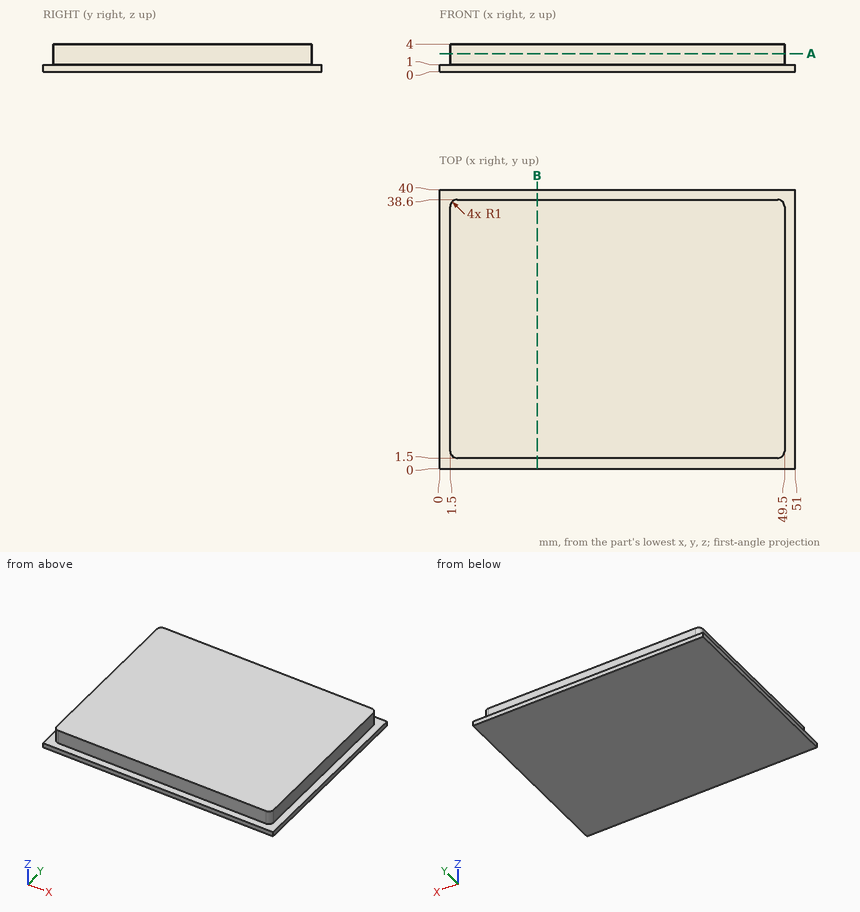
Answer from the drawing. Dimensions are ordinates in mm from the lowest x, y and z of the part. Coordinates: 2 decimals unless noted, no trailing zeros. Loops run counter-clockwise (first coordinate to the right, second up) from the corner with the lowest first, then second, coordinate; pieces in that order, holes last. Notation, with made-up numbers: (22.5, 64.25) - (67.5, 64.25) arc R21 cw to (67.5, 71.25) - close; hole circle Ø6 at (-10.75, -19). An arc over 180 degrees is marked (long way). Use a Markdown table: item, result.
Item 1: Consider probe 1 along X at (y, z) = (13, 2.8); probe 2 along Y at (x, z) = (18, 1.25). Determine where each line is inside the solid, lowest interval first. Write a range as from..to.
Evaluation:
| item | result |
|---|---|
| probe 1 | x = 1.5..49.5 |
| probe 2 | y = 1.5..38.6 |
Item 2: Find section A-A, the plane z = 2.6. Determine the outline of the cut face in (x, y), and give its area (3 significant figures).
Evaluation:
| item | result |
|---|---|
| outline | (1.5, 2.5) arc R1 ccw to (2.5, 1.5) - (48.5, 1.5) arc R1 ccw to (49.5, 2.5) - (49.5, 37.6) arc R1 ccw to (48.5, 38.6) - (2.5, 38.6) arc R1 ccw to (1.5, 37.6) - close |
| area | 1,780 mm2 |
Item 3: Find section B-B, the plane x = 14. Determine the outline of the cut face in (y, z).
Evaluation:
| item | result |
|---|---|
| outline | (0, 0) - (40, 0) - (40, 1) - (38.6, 1) - (38.6, 4) - (1.5, 4) - (1.5, 1) - (0, 1) - close |
Item 4: Given pin 1 Ø0.9 at (x, z) = (30.5, 2.5) entering from +Y; pin 2 Ø1.5 at (y, z) = (22.5, 2.5) entering from -X, each flat-ended and moving along its own axis, determine where each tip first touches the part or whether it passes through.
Evaluation:
| item | result |
|---|---|
| pin 1 | stops at y = 38.6 |
| pin 2 | stops at x = 1.5 |
